Geometry: see drawing. Coordinates: mm, zero at the bounding-box minimum. Round coordinates to 2 decimals unless told otherwise and drop trailing zeros. Loops run counter-clockwise (first coordinate to the right, second up) from the corner with the lowest first, then second, coordinate; pieces in that order, holes last. Notation, with made-up numbers: (-38.75, 11) - (-19.75, 11) arc R31 cw to (-19.75, 39) - close; hole circle Ø4 at (63, -6). An arc over 180 degrees is marked (long way). Return JSON: item names as keys, results as strings. Group by question number.
1. First-contact query: pin 1 Ø2.5 at (y, z) = (137, 2.5) entering from +X; pin 2 Ø1.5 at (y, z) = (4, 3.5) entering from -X; pin 3 Ø3 at (x, z) = (57.5, 1.5) entering from -Y. Flat tips, straight axial feed; report the tip coordinate or a pass-through.
2. Material intervals for probe 1 along X at (y, z) = (7, 0.25); probe 2 along Y at (x, z) = (18, 4.3), sorted ascending.
3. Section A-A on x = 126.5. Return loops of the section in (y, z).
4. Draft query along Z for the marked faces 1 and 2. Return one class per face: +Z half, -Z half, draft (parallel to the pull), parting line (faces both ways), or undercut.
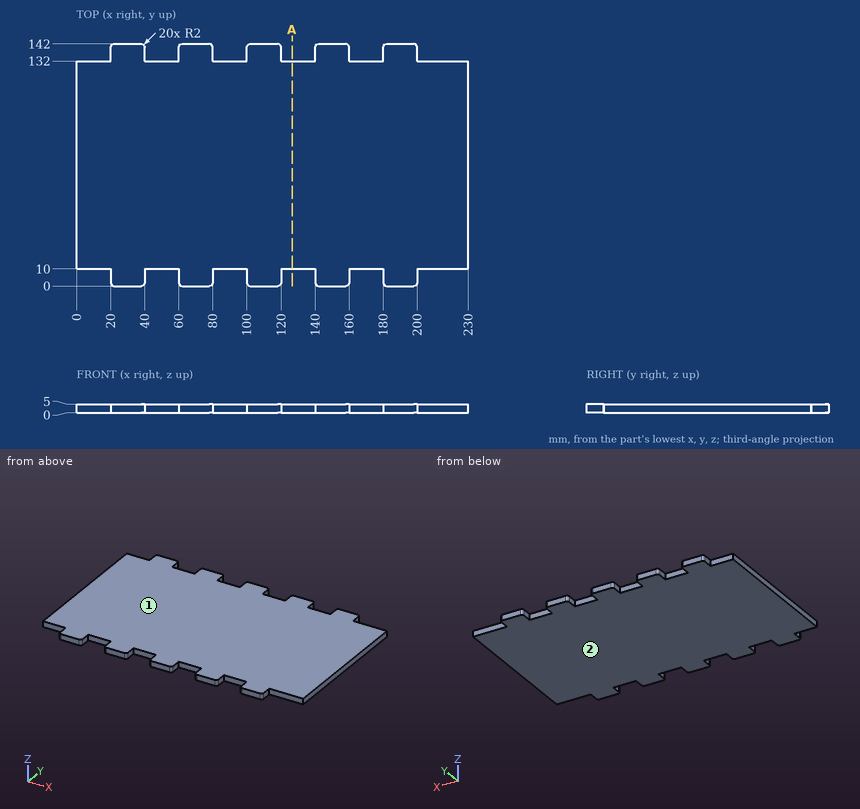
Taken from the geometry:
{
 "1": {"pin 1": "x = 200", "pin 2": "x = 20", "pin 3": "y = 10"},
 "2": {"probe 1": "20 to 40, 60 to 80, 100 to 120, 140 to 160, 180 to 200", "probe 2": "10 to 132"},
 "3": {"outline": "(10, 0) - (132, 0) - (132, 5) - (10, 5) - close"},
 "4": {"face 1": "+Z half", "face 2": "-Z half"}
}
